Input: dimensioned drawing with shaded views. Units: mm. Origin: part minimum x, y, z. A direction names the side the tool comes from. Round coordinates to 2 decimals unless told otherwise and drop trailing zeros. Order: outer loops, then holes, each group sorted by start corner. A loop starts at its lowest first (then second) coordinate and runs counter-clockwise, first axis right, second up. Notation, with made-up numbers: (5, 1) - (36, 1) arc R29 cw to (36, 33) - close; hole circle Ø1 at (13, 18.25). An arc over 180 degrees is marked (long way). Put each result on its own line as item: value. Start each with the question number.
(1) Section A-A (x = 1.75). Output: boundary loops of the cut face in (y, z) (3 decimals), and give its area (3 significant figures).
(2) Section C-C (z = 4.5). Output: boundary loops of the cut face in (x, y) (3 decimals), and give its area (3 significant figures).
(3) Access query for the marked faces 4 and 5. Directions: +Z, -Z, +X, -X, +Y, -Y. A direction counts if a zero-diameter tool reaches every point of the face in a straight line with its end or side. Return the directions, or none.
(4) Section B-B (y = 44). Output: boundary loops of the cut face in (x, z), and give its area (3 significant figures).
(5) Pull-direction query (X, two-part tool) for the marked faces 1, 2 and 3; classes: released by +X, released by -X, zero draft, split by the parting line, or undercut.
(6) Material intervals for L1, parallel to Z at x = 2.5, y = 31; L2, parallel to X at y = 34.5, z = 36; L3, parallel to Z at x = 8.25, y = 45.5, sorted ascending. Write a range as [from, to].
(7) Pin query (flat end, axial travel): P1, Ø4, axis at y = 13, z = 15.5, coming from the -X side. Return the tip coordinate at first contact, or that it passes through.
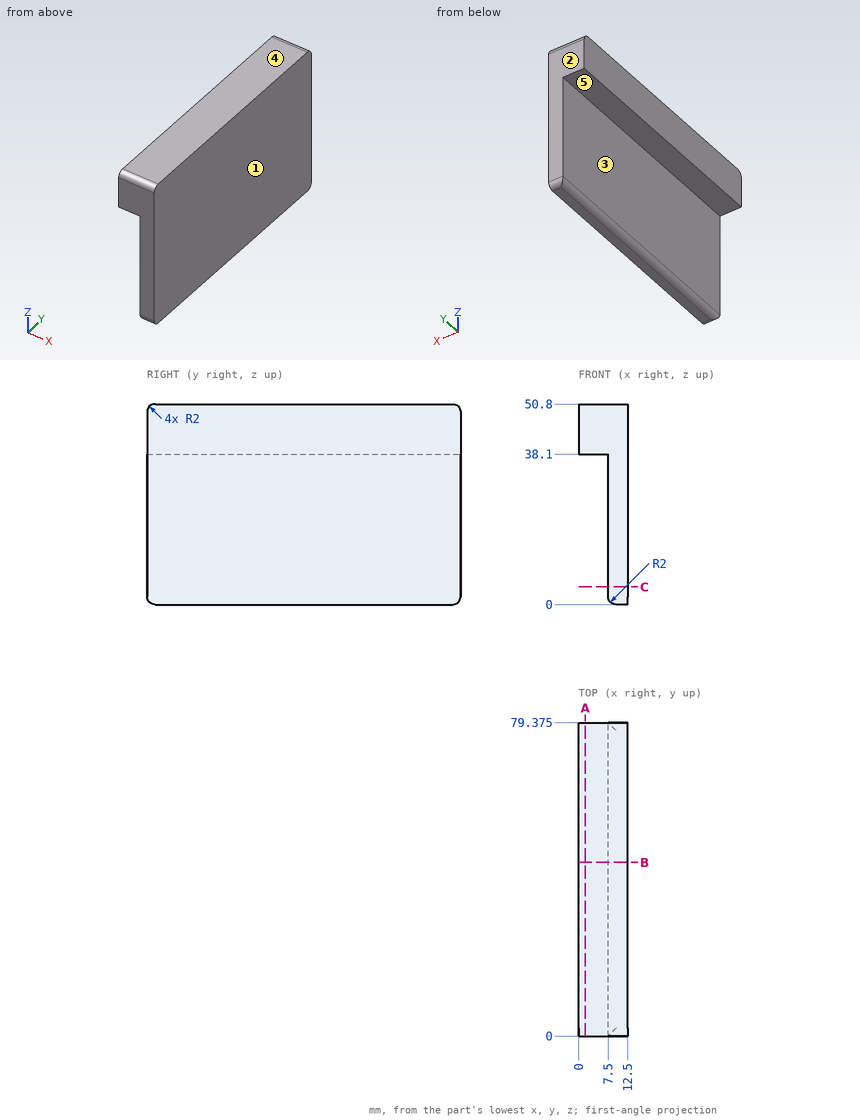
Checks:
1. outline: (0, 38.1) - (79.375, 38.1) - (79.375, 48.8) arc R2 ccw to (77.375, 50.8) - (2, 50.8) arc R2 ccw to (0, 48.8) - close
1. area: 1,010 mm²
2. outline: (7.5, 0) - (12.5, 0) - (12.5, 79.375) - (7.5, 79.375) - close
2. area: 397 mm²
3. face 4: +Z, +X, -X, +Y, -Y
3. face 5: -Z, -X, +Y, -Y
4. outline: (0, 38.1) - (7.5, 38.1) - (7.5, 2) arc R2 ccw to (9.5, 0) - (12.5, 0) - (12.5, 50.8) - (0, 50.8) - close
4. area: 348 mm²
5. face 1: released by +X
5. face 2: zero draft
5. face 3: released by -X
6. L1: z = [38.1, 50.8]
6. L2: x = [7.5, 12.5]
6. L3: z = [0.44, 50.8]
7. P1: stops at x = 7.5
